Job drawing, mm, ordinate dimensions from the low corner. One solid piece. Round coordinates to 2 decimals unless told otherwise and drop trailing zeros. Loops run counter-clockwise (first coordinate to the right, second up) from the corner with the lowest first, then second, coordinate; pieces in that order, holes last.
1) Probe line 1 (Y direction, x = 2.7, z = 1.8); line 2 (X direction, y = 70.05, z = 1.7); line 3 (X direction, y = 12, z = 4.4). List the from-to ranges inside material, lowest first.
2) Band-saw the part on B-B, the plane y = 38. Write the cut outline in (x, z).
3) Band-saw the part on D-D, the plane z = 0.95. Write the cut outline in (x, y), then the cut area to 3 significant figures.
4) Band-saw the part on C-C, the plane x = 2.7. Write the cut outline in (y, z), then the cut area to 3 significant figures.
5) Band-saw the part on A-A, the plane y = 22.05. Write the cut outline in (x, z).
6) Drop flat-ended pins along their axis: P1, Ø2.5, axis at x = 2.7, y = 118.049, coming from the +Z side; P2, Ø2.5, axis at x = 18, z = 1.5, coming from the -Y side. Give the stop position or say it passes through.
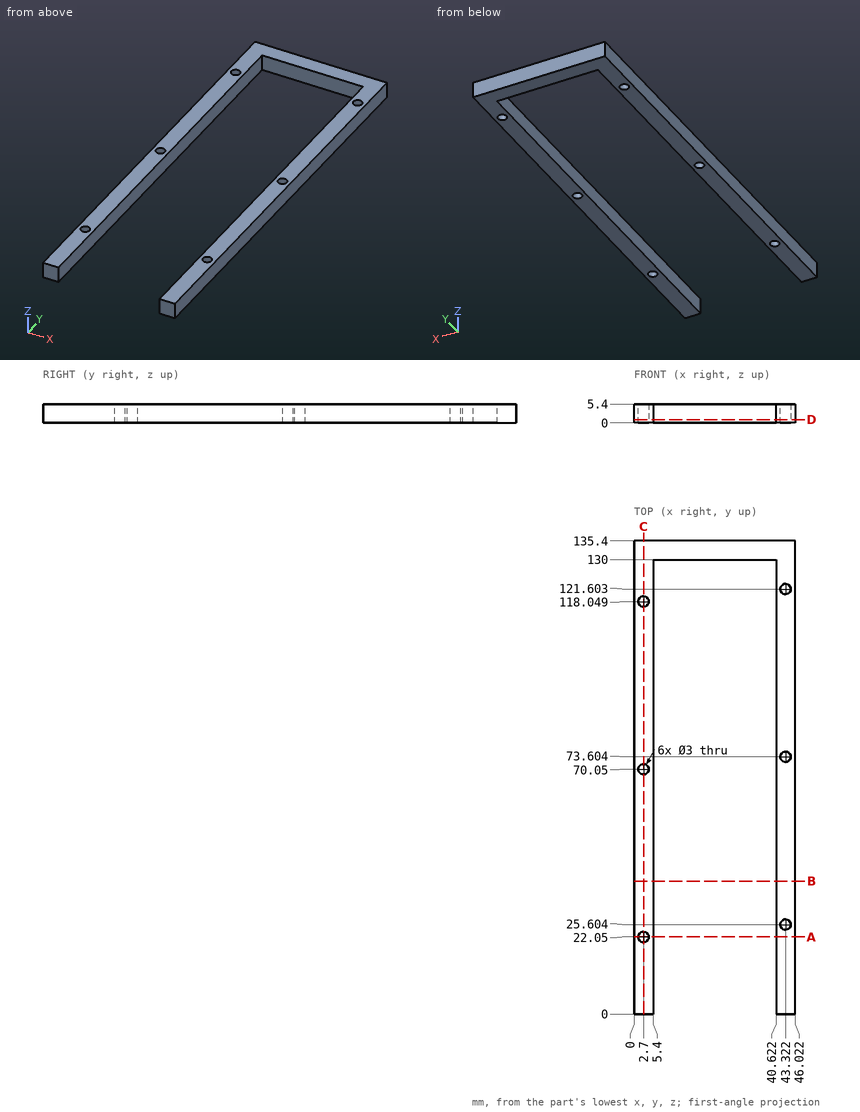
Reported:
1. line 1: y = 0 to 20.55, 23.55 to 68.55, 71.55 to 116.55, 119.55 to 135.4
1. line 2: x = 0 to 1.2, 4.2 to 5.4, 40.62 to 46.02
1. line 3: x = 0 to 5.4, 40.62 to 46.02
2. outline: (0, 0) - (5.4, 0) - (5.4, 5.4) - (0, 5.4) - close; (40.62, 0) - (46.02, 0) - (46.02, 5.4) - (40.62, 5.4) - close
3. outline: (0, 0) - (5.4, 0) - (5.4, 130) - (40.62, 130) - (40.62, 0) - (46.02, 0) - (46.02, 135.4) - (0, 135.4) - close; hole circle Ø3 at (2.7, 22.05); hole circle Ø3 at (2.7, 70.05); hole circle Ø3 at (2.7, 118.05); hole circle Ø3 at (43.32, 25.6); hole circle Ø3 at (43.32, 73.6); hole circle Ø3 at (43.32, 121.6)
3. area: 1,610 mm2
4. outline: (0, 0) - (20.55, 0) - (20.55, 5.4) - (0, 5.4) - close; (23.55, 0) - (68.55, 0) - (68.55, 5.4) - (23.55, 5.4) - close; (71.55, 0) - (116.55, 0) - (116.55, 5.4) - (71.55, 5.4) - close; (119.55, 0) - (135.4, 0) - (135.4, 5.4) - (119.55, 5.4) - close
4. area: 683 mm2
5. outline: (0, 0) - (1.2, 0) - (1.2, 5.4) - (0, 5.4) - close; (4.2, 0) - (5.4, 0) - (5.4, 5.4) - (4.2, 5.4) - close; (40.62, 0) - (46.02, 0) - (46.02, 5.4) - (40.62, 5.4) - close
6. P1: passes through
6. P2: stops at y = 130
